Design review of the part built by this model. Coordinates are the model's own, in mm. A direction names the side the tool comes from. Round coordinates to 2 decimals unless told otherwise and drop trailing zeros. Loops run counter-clockwise (first coordinate to the right, second up) from the corner with the lowest first, then second, coordinate; pieces in that order, holes last. Notation, with made-up numbers: M 63,34.25 L 87,34.25 A26 cw 87,65.25 Z; hole C 27.5,51.25 d1. An arc over 180 degrees is marked long. Use a Markdown table: item, result.
from build123d import *

# Parameters (mm, degrees)
F0_R        = 25
F0_R_2      = 18.25
F1_DEPTH    = 54
F4_D        = 8.8
F4_DEPTH    = 15.75
F4_START    = 1.3902459
F4_TIP      = 2.6437867237
F5_R        = 32.5
F6_DEPTH    = 80
F7_R        = 24.25
F8_DEPTH    = 70
F9_S5_R     = 25
F9_T6_DEPTH = 48
F12_D       = 8.8


# Not quite as in the source:
# - a fillet or chamfer that OpenCascade refuses, or shapes differently, is made with other operations: its cross-section is extruded or revolved along the edge and cut away or added


with BuildPart() as f1:
    # F0 (on Top) → F1 (new body)
    with BuildSketch(Plane.XY):
        Circle(F0_R)
        Circle(F0_R_2, mode=Mode.SUBTRACT)
    extrude(amount=F1_DEPTH)

    # F4
    # its depths count from where the whole tool has entered the part; down to there all is cleared
    with Locations(Plane.XZ.offset(26).offset(-F4_START)):
        with Locations((0, 10), (0, 30)):
            Hole(F4_D / 2, depth=F4_DEPTH)
            with Locations((0, 0, -(F4_DEPTH + F4_TIP / 2))):  # 118° drill point
                Cone(0, F4_D / 2, F4_TIP, mode=Mode.SUBTRACT)

    # F5 (on face) → F6 (join)
    with BuildSketch(Plane.XY):
        Circle(F5_R)
    extrude(amount=-F6_DEPTH)

    # F7 (on face) → F8 (cut)
    with BuildSketch(Plane(origin=(0, 0, -80), x_dir=(1, 0, 0), z_dir=(0, 0, -1))):
        Circle(F7_R)
    extrude(amount=-F8_DEPTH, mode=Mode.SUBTRACT)

    # F9: chamfer of 8 on 1 edges, made by hand


with BuildPart() as f9_tool2:
    # F9_s3 → F9_t4 (revolve)
    with BuildSketch(Plane.XZ):
        Polygon((32.5, -8), (24.5, 0), (32.5, 0), align=None)
    revolve(axis=Axis((0, 0, 0), (0, 0, 1)))

    # F9_s5 → F9_t6 (cut, symmetric)
    with BuildSketch(Plane.XY.offset(-4)):
        Circle(F9_S5_R)
    extrude(amount=F9_T6_DEPTH, both=True, mode=Mode.SUBTRACT)


with BuildPart() as f1_1:
    add(f1.part)

    # F9_t1: cut F9_tool2
    add(f9_tool2.part, mode=Mode.SUBTRACT)

    # F12 (through all)
    with Locations(Plane.XZ.offset(51)):
        with Locations((0, -33), (0, -65)):
            Hole(F12_D / 2)


solid = f1_1.part
1. Take a section at D-D on z = -31.5. Give the boundary of the cut face in (x, y), and give its area (3 significant figures).
Check values:
| item | result |
|---|---|
| outline | M -4.14,-32.24 L -4.14,-23.89 A24.25 cw -4.14,23.89 L -4.14,32.24 A32.5 ccw Z; M 4.14,-32.24 A32.5 ccw 4.14,32.24 L 4.14,23.89 A24.25 cw 4.14,-23.89 Z |
| area | 1,330 mm² |
2. Take a section at C-C on x = 0. Count the separate pieces of the cut face and the enclosed holes in it, and give its area (3 significant figures).
Check values:
| item | result |
|---|---|
| separate pieces | 7 |
| enclosed holes | 0 |
| area | 2,060 mm² |
3. The part is to be moulded in two halves that separate along X. For faces 1 (the face through (-12, -22, -80)), 2 (the face through (31, 9.76, -43.5)), 3 (the face through (0, 0, 0)), say which applies: pulls with the +X half, pulls with the -X half, needs draft (parallel to the pull), parting line crosses it, or undercut.
Check values:
| item | result |
|---|---|
| face 1 | needs draft |
| face 2 | parting line crosses it |
| face 3 | undercut |
4. Take a section at A-A on z = -65. Give the boundary of the cut face in (x, y), and give its area (3 significant figures).
Check values:
| item | result |
|---|---|
| outline | M -4.4,-32.2 L -4.4,-23.85 A24.25 cw -4.4,23.85 L -4.4,32.2 A32.5 ccw Z; M 4.4,-32.2 A32.5 ccw 4.4,32.2 L 4.4,23.85 A24.25 cw 4.4,-23.85 Z |
| area | 1,330 mm² |
5. Machinability: for faces 4 (the face through (1.7, -18.4, 54)), 5 (the face through (0, 0, -10)), 6 (the face through (0.954, 28.233, -69.295)), 7 (the face through (4.396, -21.303, 10.193)), 8 (the face through (9.81, 15.39, 26.62)), which of the approach directions +Z, -Z, +X, -X, +Y, -Y give a long, thin tool a straight path to every point of the face, cutting with its end or side? Answer none if there is none.
Check values:
| item | result |
|---|---|
| face 4 | +Z, +X, -X, +Y, -Y |
| face 5 | -Z |
| face 6 | +Y, -Y |
| face 7 | -Y |
| face 8 | +Z |
6. Take a section at B-B on y = 0. Give the boundary of the cut face in (x, z).
Check values:
| item | result |
|---|---|
| outline | M -32.5,-80 L -24.25,-80 L -24.25,-10 L 24.25,-10 L 24.25,-80 L 32.5,-80 L 32.5,-8 L 25,-0.5 L 25,54 L 18.25,54 L 18.25,0 L -18.25,0 L -18.25,54 L -25,54 L -25,-0.5 L -32.5,-8 Z |
7. Insertion check: pin 1 (1.5 mm diameter, centred on x = -8.5, y = 6, fed in from +Z); pin 2 (4 mm diameter, centred on x = 3, y = 13, fed in from -Z); pin 3 (5 mm diameter, centred on y = -8.5, z = -61.5, fed in from +X). Each pin has a flat end and moves straight along its axis. Give the tip position at first contact, or say it passes through.
Check values:
| item | result |
|---|---|
| pin 1 | stops at z = 0 |
| pin 2 | stops at z = -10 |
| pin 3 | stops at x = 31.94 |
8. Wall thickness on line 1 along Z through (x, y) = (0, 30); line 2 along Z through (x, y) = (-12, -10.5); line 3 along Y through (x, z) = (0, 34): over which ranges is each line inside the solid? List them lowest first. Write a range as from..to.
Check values:
| item | result |
|---|---|
| line 1 | z = -80..-69.4, -60.6..-37.4, -28.6..-5.5 |
| line 2 | z = -10..0 |
| line 3 | y = 18.25..25 |
